Can you work these out from the model? Positions are in its coordinate system, mm. A direction names the side the tool comes from. Give positions to 0.01 mm unless a question says otherwise; leave off trailing zeros. Loops run counter-clockwise (first coordinate to the right, second up) from the corner with the lowest first, then second, coordinate; pieces in that order, holes last. Notation, with made-up numbers: (-20.5, 38.25) -> (16.5, 38.25) arc R31 ccw to (16.5, 71.25) -> close; hole circle Ø9 at (4, 82). An arc over 180 degrees is marked (long way). Return JSON: item names as keys, results as strings. Group by question number.
Q1. Will these pins go through, and if not, where does the flat tip stop? pin 1 (3.5 mm diameter, centred on x = 15, z = 0, fed in from -Y); pin 2 (4.5 mm diameter, centred on x = -15, z = 0, fed in from +Y); pin 3 (9 mm diameter, centred on x = -16, y = 13, fed in from +Z); pin 4 (8 mm diameter, centred on y = 14.5, z = 21.5, fed in from -X).
Q2. Suppose I cut it at B-B, the plane z = 0. Please give me the cut outline in (x, y).
Q3. I need wall thicknesses on line 1 along Z through (x, y) = (15, 13); line 2 along X through (y, z) = (5.25, -11.5); line 3 along Z through (x, y) = (-14.5, 9.25). Which ranges of each line are inside material? Lowest first, please. Write a range as [from, to].
Q4. Which directions (+Z, -Z, +X, -X, +Y, -Y) give clear straight access to the entire face, cutting with the end or side of a thin tool? Please do faces 4 (the flat face through (-44.9, 9, 35)), 5 (the flat face through (-7, 9, 35.4)), 6 (the flat face through (-26.1, 9, -4)).
Q5. Suppose I cut it at C-C, the plane x = 15. Please give me the cut outline in (y, z).
Q6. Suppose I cut it at A-A, the plane y = 7. Please give me the cut outline in (x, z).
Q7. Suppose I cut it at D-D, the plane z = 16. Please give me the cut outline in (x, y).
Q8. Thinking about a two-plate mould opening in X: for faces 1 (the flat face through (-2, 0, 2)), 2 (the flat face through (-35.62, 8.73, 28.83)), 3 (the cylindrical face through (-16.6, 8.7, -1.2)), which applies, pulls with the +X half, pulls with the -X half, needs draft (parallel to the pull), parting line crosses it, or undercut?
```python
from build123d import *

# Parameters (mm, degrees)
F0_R        = 2
F1_DEPTH    = 17.7
F2_T1_DEPTH = 25.2
F2_T3_DEPTH = 23.679138459
F3_R        = 0.8


# Not quite as in the source:
# - a fillet or chamfer that OpenCascade refuses, or shapes differently, is made with other operations: its cross-section is extruded or revolved along the edge and cut away or added


with BuildPart() as f1:
    # F0 (on Front) → F1 (new body)
    with BuildSketch(Plane.XZ):
        Polygon((26.1, 35.4), (-41.5, 35.4), (-42.3, 38.9), (-44.9, 38.9), (-44.9, 31.2), (-26.1, 26.4), (-26.1, -35.4), (26.1, -35.4), align=None)
        with Locations((-15, 0)):
            Circle(F0_R, mode=Mode.SUBTRACT)
        with Locations((15, 0)):
            Circle(F0_R, mode=Mode.SUBTRACT)
    extrude(amount=-F1_DEPTH)

    # F2: fillet of radius 1.5 on 2 edges, made by hand

    # F2_s2 → F2_t1 (cut)
    with BuildSketch(Plane.XZ.offset(-21.45)):
        with BuildLine():
            ThreePointArc((-43.4, 38.9), (-44.4606601718, 38.4606601718), (-44.9, 37.4))
            Line((-44.9, 37.4), (-44.9, 38.9))
            Line((-44.9, 38.9), (-43.4, 38.9))
        make_face()
    extrude(amount=F2_T1_DEPTH, mode=Mode.SUBTRACT)

    # F2_s4 → F2_t3 (cut)
    with BuildSketch(Plane.XZ.offset(-20.6895692295)):
        with BuildLine():
            ThreePointArc((-42.0335399319, 37.7342372023), (-42.560775769, 38.5728929626), (-43.4958276918, 38.9))
            Line((-43.4958276918, 38.9), (-42.3, 38.9))
            Line((-42.3, 38.9), (-42.0335399319, 37.7342372023))
        make_face()
    extrude(amount=F2_T3_DEPTH, mode=Mode.SUBTRACT)

    # F3
    f3_edges = [f1.edges().sort_by_distance(p)[0] for p in [
        (-41.5, 8.85, 35.4),
        (26.1, 8.85, 35.4),
        (26.1, 8.85, -35.4),
        (-44.9, 8.85, 31.2),
        (-26.1, 8.85, 26.4),
        (-26.1, 8.85, -35.4),
    ]]
    fillet(f3_edges, radius=F3_R)


solid = f1.part
```
Ans:
{
 "1": {"pin 1": "passes through", "pin 2": "stops at y = 17.7", "pin 3": "stops at z = 35.4", "pin 4": "stops at x = -26.1"},
 "2": {"outline": "(-26.1, 0) -> (-17, 0) -> (-17, 17.7) -> (-26.1, 17.7) -> close; (-13, 0) -> (13, 0) -> (13, 17.7) -> (-13, 17.7) -> close; (17, 0) -> (26.1, 0) -> (26.1, 17.7) -> (17, 17.7) -> close"},
 "3": {"line 1": "z = [-35.4, -2], [2, 35.4]", "line 2": "x = [-26.1, 26.1]", "line 3": "z = [-35.4, -1.94], [1.94, 35.4]"},
 "4": {"face 4": "+Z, -Z, -X, +Y, -Y", "face 5": "+Z, +X, +Y, -Y", "face 6": "-Z, -X, +Y, -Y"},
 "5": {"outline": "(0, -35.4) -> (17.7, -35.4) -> (17.7, -2) -> (0, -2) -> close; (0, 2) -> (17.7, 2) -> (17.7, 35.4) -> (0, 35.4) -> close"},
 "6": {"outline": "(-44.9, 31.82) arc R0.8 ccw to (-44.3, 31.05) -> (-26.7, 26.55) arc R0.8 cw to (-26.1, 25.78) -> (-26.1, -34.6) arc R0.8 ccw to (-25.3, -35.4) -> (25.3, -35.4) arc R0.8 ccw to (26.1, -34.6) -> (26.1, 34.6) arc R0.8 ccw to (25.3, 35.4) -> (-40.86, 35.4) arc R0.8 cw to (-41.64, 36.02) -> (-42.03, 37.73) arc R1.5 ccw to (-43.45, 38.9) arc R1.5 ccw to (-44.9, 37.4) -> close; hole circle Ø4 at (-15, 0); hole circle Ø4 at (15, 0)"},
 "7": {"outline": "(-26.1, 0) -> (26.1, 0) -> (26.1, 17.7) -> (-26.1, 17.7) -> close"},
 "8": {"face 1": "needs draft", "face 2": "pulls with the -X half", "face 3": "undercut"}
}
